from build123d import *

# Parameters (mm, degrees)
SKETCH_1_R      = 2
SKETCH_1_R_2    = 1
EXTRUDE_1_DEPTH = 225


with BuildPart() as part:
    # 草圖1 → 填料-伸長1 (new, symmetric)
    with BuildSketch(Plane(origin=(0, 0, 0), x_dir=(1, 0, 0), z_dir=(0, 1, 0))):
        Polygon((-10, -10), (-2, -10), (-2, -9), (-3, -9), (-3, -7), (-2, -6), (2, -6), (3, -7), (3, -9), (2, -9), (2, -10), (10, -10), (10, -2), (9, -2), (9, -3), (7, -3), (6, -2), (6, 2), (7, 3), (9, 3), (9, 2), (10, 2), (10, 10), (2, 10), (2, 9), (3, 9), (3, 7), (2, 6), (-2, 6), (-3, 7), (-3, 9), (-2, 9), (-2, 10), (-10, 10), (-10, 2), (-9, 2), (-9, 3), (-7, 3), (-6, 2), (-6, -2), (-7, -3), (-9, -3), (-9, -2), (-10, -2), align=None)
        with Locations(Location((0, 0, 0), (0, 0, 270))):
            Circle(SKETCH_1_R, mode=Mode.SUBTRACT)
        with Locations(Location((-7, 7, 0), (0, 0, 270))):
            Circle(SKETCH_1_R_2, mode=Mode.SUBTRACT)
        with Locations(Location((7, 7, 0), (0, 0, 270))):
            Circle(SKETCH_1_R_2, mode=Mode.SUBTRACT)
        with Locations(Location((7, -7, 0), (0, 0, 270))):
            Circle(SKETCH_1_R_2, mode=Mode.SUBTRACT)
        with Locations(Location((-7, -7, 0), (0, 0, 270))):
            Circle(SKETCH_1_R_2, mode=Mode.SUBTRACT)
    extrude(amount=EXTRUDE_1_DEPTH, both=True)


solid = part.part
Work out the finished part from the listing and answer in its coordinate system (mm). Give positions to 0.01 mm unless a question says otherwise; leave off trailing zeros. Return JSON: item names as keys, results as strings.
Q1. Find the intervals of material crossed by line 1 along X through (y, z) = (131.5, 7); line 2 along X through (y, z) = (24.5, -8.5); line 3 along Z through (x, y) = (2.5, -9), in increasing order. Write a range as [from, to].
Answer below:
{"line 1": "x = [-10, -8], [-6, -3], [3, 6], [8, 10]", "line 2": "x = [-10, -3], [3, 10]", "line 3": "z = [-10, -9], [-6.5, 6.5], [9, 10]"}
Q2. Find section A-A, the plane y = 106. State how many separate pieces and enclosed holes the cut face has, and give its area (3 significant figures).
Answer below:
{"separate pieces": "1", "enclosed holes": "5", "area": "291 mm^2"}
Q3. Each of these flat-tipped pins is pushed along its axis until it touches: pin 1 (1.2 mm diameter, centred on y = -62.5, z = 1, fed in from -X); pin 2 (1.2 mm diameter, centred on x = 0.5, y = -109, fed in from +Z); pin 3 (1.2 mm diameter, centred on y = -53, z = -0.5, fed in from +X). Where does it stop, or does it pass through?
Answer below:
{"pin 1": "stops at x = -6", "pin 2": "stops at z = 6", "pin 3": "stops at x = 6"}
